Autodesk Inventor part; units mm, degrees
ref_plane "YZ Plane" through (0, 0, 0) normal (1, 0, 0) x (0, 1, 0)
ref_plane "XZ Plane" through (0, 0, 0) normal (0, 1, 0) x (-1, 0, 0)
ref_plane "XY Plane" through (0, 0, 0) normal (0, 0, 1) x (1, 0, 0)
sketch "スケッチ2" plane through (0, 0, 0) normal (0, 0, 1) x (1, 0, 0)
  line L0 (0, 0) -> (26, 0)
  line L1 (26, 0) -> (26, 33)
  line L2 (26, 33) -> (0, 33)
  line L3 (0, 33) -> (0, 0)
  line L4 (0, 0) -> (26, 0)
  line L5 (26, 0) -> (26, 24)
  line L6 (26, 24) -> (0, 24) construction
  line L7 (0, 24) -> (0, 0)
  circle A0 centre (13, 24) radius 13
  circle A1 centre (13, 24) radius 6.25
  line L8 (26, 0) -> (0, 0)
  line L9 (26, 24.5219) -> (26, -21)
  line L10 (26, -21) -> (0, -21)
  line L11 (0, -21) -> (0, 24)
  circle A2 centre (5, -19) radius 0.8
  circle A3 centre (21, -19) radius 0.8
  line L12 (0, 24) -> (26, 24)
  point P0 (22.3808, 33)
  point P1 (3.6192, 33)
  point P2 (0, 0)
  point P3 (26, 24)
  point P4 (0, 24)
  point P5 (6.75, 24)
  point P6 (19, 22.25)
  point P7 (19.25, 24)
  dimension "d0" = 26
  dimension "d1" = 33
  dimension "d2" = 24
  dimension "d3" = 12.5
  dimension "d14" = 26
  dimension "d17" = 1.6
  dimension "d18" = 1.6
  dimension "d19" = 2
  dimension "d20" = 2
  dimension "d21" = 5
  dimension "d22" = 5
  dimension "d23" = 13
  dimension "d25" = 45
  dimension "d26" = 0
extrude "押し出し1" add sketch "スケッチ2" along normal blind 1.5 contours L3 A0 L1 L0 | L0 L9 L10 L11 | L12 A1 A0 | A0 L2 L12 A1 | A0 L2 L1 | L12 A1 | A1 L12
sketch "スケッチ3" plane through (0, 0, 0) normal (0, 0, -1) x (-1, 0, 0)
  circle A0 centre (-2.5, 24) radius 0.85
  circle A1 centre (-23.5, 24) radius 0.85
  circle A2 centre (-23.5, 3) radius 0.85
  circle A3 centre (-2.5, 3) radius 0.85
  circle A4 centre (-13, 24) radius 6.25
  line L0 (-2.5, 24) -> (-23.5, 24)
  line L1 (-23.5, 24) -> (-23.5, 3)
  line L2 (-23.5, 3) -> (-2.5, 3)
  line L3 (-2.5, 3) -> (-2.5, 24)
  circle A5 centre (-13, 24) radius 10.25
  line L4 (-5.5, 24) -> (-20.5, 24)
  line L5 (-20.5, 24) -> (-20.5, 3)
  line L6 (-20.5, 3) -> (-5.5, 3)
  line L7 (-5.5, 3) -> (-5.5, 24)
  arc A6 (0, 24) -> (-3.6192, 33) centre (-13, 24) ccw
  line L8 (-26, 33) -> (-3.6192, 33)
  line L9 (-26, -21) -> (-26, 33)
  line L10 (0, -21) -> (-26, -21)
  line L11 (0, 24) -> (0, -21)
  circle A7 centre (-5, -19) radius 0.8
  circle A8 centre (-21, -19) radius 0.8
  line L12 (-37.149, 0) -> (-22.2321, 0)
  line L13 (-22.2321, 0) -> (-8, 0)
  circle A9 centre (-23.5, 3) radius 2.5
  circle A10 centre (-2.5, 3) radius 2.5
  line L14 (-21.5265, 4.5347) -> (-18, 0)
  line L15 (-4.4735, 4.5347) -> (-8, 0)
  line L16 (-18, 0) -> (-8, 0)
  circle A11 centre (-21, -19) radius 2
  circle A12 centre (-5, -19) radius 2
  line L17 (-26, -21) -> (-26, 33)
  line L18 (-19.4, -20.2) -> (-17, -17)
  line L19 (-17, -17) -> (-9, -17)
  line L20 (-9, -17) -> (-6.6, -20.2)
  line L21 (-25.977, 2.6617) -> (-22.9816, -19.2706)
  line L22 (-0.023, 2.6617) -> (-3.0184, -19.2706)
  line L23 (-23.5, 3) -> (-21, -19)
  line L24 (-2.5, 3) -> (-5, -19)
  line L25 (-23.1591, 0) -> (-2.8409, 0)
  line L26 (-21.5682, -14) -> (-4.4318, -14)
  line L27 (-21.1462, 0) -> (-19.5553, -14)
  line L28 (-4.8538, 0) -> (-6.4447, -14)
  point P0 (0, 0)
  point P1 (-5.5, 17.0134)
  point P2 (-20.5, 17.0134)
  point P3 (-13, 0)
  point P4 (-13, -21)
  point P5 (-13, -17)
  point P6 (-21, -21)
  point P7 (-5, -21)
  point P8 (-25.6135, 0)
  point P9 (-26, 0)
  point P10 (0, 3)
  point P11 (-8.0946, 33)
  point P12 (-17.9054, 33)
  point P13 (-26, 3)
  point P14 (-20.5, 3.2147)
  point P15 (-5.5, 3.2147)
  point P16 (-3.35, 3)
  point P17 (-2.5, 3.85)
  point P18 (-2.5, 5.5)
  point P19 (-23.5, 5.5)
  point P20 (-23.5, 3.85)
  point P21 (-22.65, 3)
  point P22 (-5.667, 3)
  point P23 (-20.333, 3)
  dimension "d27" = 4
  dimension "d28" = 3
  dimension "d29" = 3
  dimension "d36" = 3
  dimension "d38" = 10
  dimension "d39" = 8
  dimension "d40" = 3
  dimension "d41" = 3
  dimension "d42" = 2
  dimension "d43" = 2
extrude "押し出し2" cut sketch "スケッチ3" against normal through all contours A0 L3 L0 A5 | A0 A5 L8 A6 L11 A10 L3 | A5 L0 A0 | A0 L0 A4 A1 A5 L8 | L3 A10 L15 L7 A5 A0 | A0 A5 L0 L3 | L0 A5 A0 | A0 A5 L7 L0 | L8 A5 | L7 A5 L5 L0 A4 | A5 A1 L1 A9 L9 L8 | L7 L15 L2 L14 L5 A5 | L3 L2 A3 | A3 L24 L3 | L11 L10 A12 L22 A10 | L0 A4 | A4 L0 | A5 L0 L1 A1 | A1 L0 A5 | L5 L14 A9 L1 A1 A5 | A5 A1 L0 L5 | L2 L24 A3 | A1 A5 L0 | L1 L0 A5 A1 | A9 L21 L12 L9 | L10 A11 L18 L19 L20 A12 | L12 L21 A11 L10 L9 | L25 L28 L26 L27 L13 | L1 L23 A2 | A2 L2 L1 | A2 L23 L2
fillet "フィレット1" radius 3 8 edges at (4.8538, 0, 0.75) (21.1462, 0, 0.75) (19.5553, -14, 0.75) (6.4447, -14, 0.75) (9, -17, 0.75) (17, -17, 0.75) (20.333, 3, 0.75) (5.667, 3, 0.75)
equation "\"d20\" = d19"
properties part number "elbow" material "アルミニウム 6061"
Model file for the job. Use its own axes, mm. A direction names the side the tool comes from. Give positions to 0.01 mm unless a question says otherwise; leave off trailing zeros. Order: outer loops, then holes, each group sorted by start corner. A loop starts at its lowest first (then second) coordinate and runs counter-clockwise, first axis right, second up. Notation, with made-up numbers: (-3.75, 18.5) -> (37.25, 18.5) arc R5 cw to (37.25, 23.5) -> close; hole circle Ø4 at (43.5, 40). An arc over 180 degrees is marked (long way). Use CSV: the item, a comma, the result in double quotes.
1. Band-saw the part on A-A, the plane z = 1.2. Give the cut face in (x, y), then the cut area to 3 significant figures.
Outcome:
outline,"(0.02, 2.66) -> (3.02, -19.27) arc R2 ccw to (6.6, -20.2) -> (8.1, -18.2) arc R3 cw to (10.5, -17) -> (15.5, -17) arc R3 cw to (17.9, -18.2) -> (19.4, -20.2) arc R2 ccw to (22.98, -19.27) -> (25.98, 2.66) arc R2.5 ccw to (21.53, 4.53) -> (21.23, 4.16) arc R3 cw to (18.87, 3) -> (7.13, 3) arc R3 cw to (4.77, 4.16) -> (4.47, 4.53) arc R2.5 ccw to start; hole circle Ø1.7 at (2.5, 3); hole circle Ø1.6 at (5, -19); hole (5.23, -3.34) -> (6.14, -11.34) arc R3 ccw to (9.12, -14) -> (16.88, -14) arc R3 ccw to (19.86, -11.34) -> (20.77, -3.34) arc R3 ccw to (17.79, 0) -> (8.21, 0) arc R3 ccw to start; hole circle Ø1.6 at (21, -19); hole circle Ø1.7 at (23.5, 3)"
area,"316 mm²"
2. Band-saw the part on D-D, the plane y = -14.5. Give the cut face in (x, z).
Outcome:
outline,"(2.37, 0) -> (23.63, 0) -> (23.63, 1.5) -> (2.37, 1.5) -> close"
3. 3-axis set-ups, long thin cutter, end or side, ignore diameter. For faces 1 (the flat face through (13, 1, 0)), 2 (the flat face through (18.66, -19.214, 0.74)), 3 (the flat face through (13, -14, 1)), 4 (the flat face through (13, 3, 1)): which of +Z, -Z, +X, -X, +Y, -Y reach the whole face in a straight line?
Outcome:
face 1,"-Z, +X, -X, +Y, -Y"
face 2,"+Z, -Z, -Y"
face 3,"+Z, -Z"
face 4,"+Z, -Z, +Y"
4. Drill centre lines: line 1 along Y through (x, z) = (15.5, 0.5); line 2 along Y through (x, z) = (18, 0.6); line 3 along X through (y, z) = (-3.25, 1.3). Where is each one in solid material? Low to high. Write a range as from..to.
Outcome:
line 1,"-17..-14, 0..3"
line 2,"-18.33..-13.78, -0.01..3"
line 3,"0.83..5.22, 20.78..25.17"
5. Drop flat-ended pins along their axis: pin 1 (1 mm diameter, centred on x = 23.5, y = 3, fed in from +Z); pin 2 (1.8 mm diameter, centred on x = 21, y = -19, fed in from -Z). Give the stop position or say it passes through.
Outcome:
pin 1,"through"
pin 2,"z = 0"
6. Band-saw the part on B-B, the plane x = 2.5. Give the cut face in (y, z).
Outcome:
outline,"(-15.47, 0) -> (2.15, 0) -> (2.15, 1.5) -> (-15.47, 1.5) -> close; (3.85, 0) -> (5.5, 0) -> (5.5, 1.5) -> (3.85, 1.5) -> close"
7. Mould opens along X. For faces 5 (the flat face through (1.5, -8.15, 0.74)), 6 (the flat face through (24.5, -8.15, 0.74)), 7 (the cylindrical face through (16.859, -17.325, 0.76)) say: +X half, -X half, draft (parallel to the pull), parting line (faces both ways), or undercut.
Outcome:
face 5,"-X half"
face 6,"+X half"
face 7,"undercut"
8. Band-saw the part on C-C, the plane y = -17.75. Give the cut face in (x, z), then the cut area to 3 significant figures.
Outcome:
outline,"(2.81, 0) -> (8.52, 0) -> (8.52, 1.5) -> (2.81, 1.5) -> close; (17.48, 0) -> (23.19, 0) -> (23.19, 1.5) -> (17.48, 1.5) -> close"
area,"17.1 mm²"
